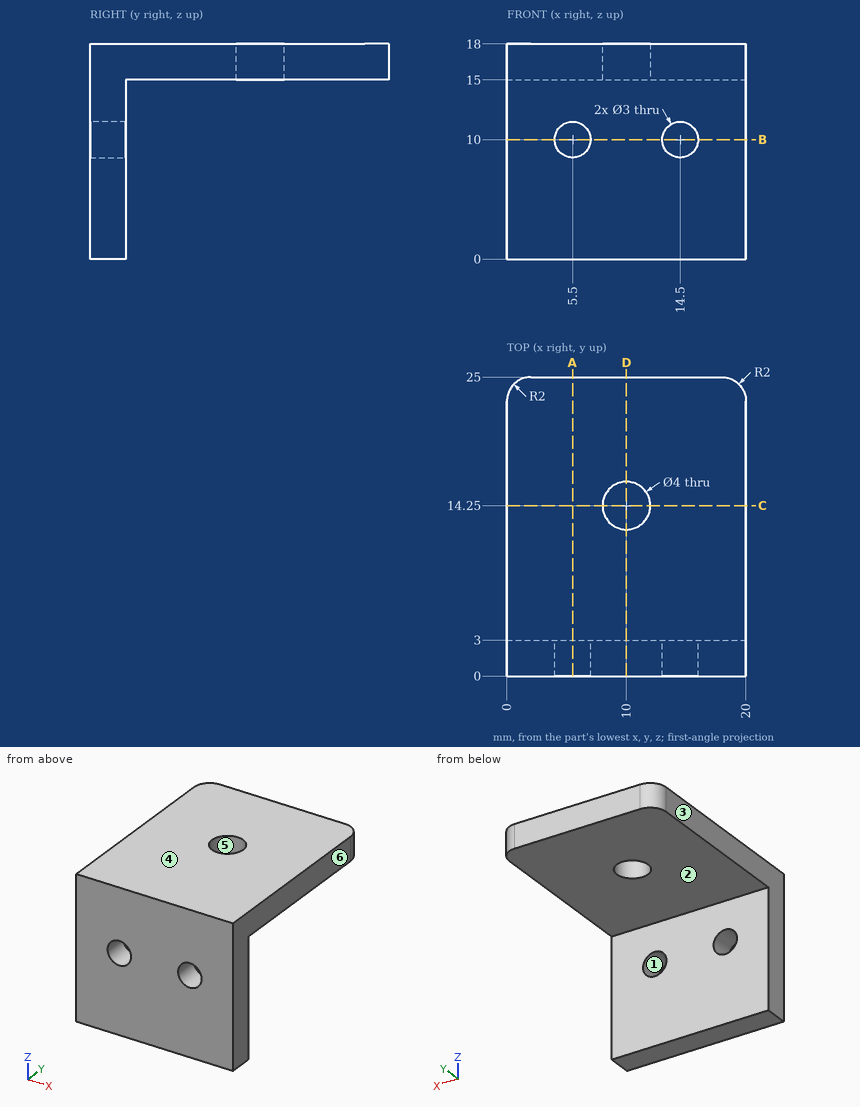
Can you work these out from the drawing? Everything is in mm from the part's minimum corner. A direction names the side the tool comes from. Round coordinates to 2 decimals unless told otherwise and drop trailing zeros. Order: outer loops, then holes, each group sorted by start corner. A loop starts at its lowest first (then second) coordinate and runs counter-clockwise, first axis right, second up. Notation, with made-up numbers: (61, -39) -> (90, -39) arc R26 cw to (90, -23) -> close; hole circle Ø10 at (1, 7). An arc over 180 degrees is marked (long way). Use CSV: the item, a comma, the result in double quotes.
1. I want a section at B-B on z = 10. List the corners of the cut face in (x, y) for me, and give its area (3 significant figures).
Recorded:
outline,"(0, 0) -> (4, 0) -> (4, 3) -> (0, 3) -> close; (7, 0) -> (13, 0) -> (13, 3) -> (7, 3) -> close; (16, 0) -> (20, 0) -> (20, 3) -> (16, 3) -> close"
area,"42.0 mm2"
2. Which directions (+Z, -Z, +X, -X, +Y, -Y) give clear straight access to the entire face, cutting with the end or side of a thin tool? Please do the marked faces 1 and 2.
Recorded:
face 1,"+Y, -Y"
face 2,"-Z, +X, -X, +Y"
3. I need wall thicknesses on line 1 along X through (y, z) = (2.25, 10); line 2 along Z through (x, y) = (16, 11.25); line 3 along Y through (x, z) = (3.75, 13.5). Which ranges of each line are inside material? Lowest first, please.
Recorded:
line 1,"x = 0 to 4, 7 to 13, 16 to 20"
line 2,"z = 15 to 18"
line 3,"y = 0 to 3"
4. I want a section at D-D on x = 10. List the corners of the cut face in (y, z) for me, and give its area (3 significant figures).
Recorded:
outline,"(0, 0) -> (3, 0) -> (3, 15) -> (12.25, 15) -> (12.25, 18) -> (0, 18) -> close; (16.25, 15) -> (25, 15) -> (25, 18) -> (16.25, 18) -> close"
area,"108 mm2"
5. Thinking about a two-plate mould opening in X: for the marked faces 3, 4, 5 and 6, which applies, pulls with the +X half, pulls with the -X half, needs draft (parallel to the pull), parting line crosses it, or undercut?
Recorded:
face 3,"pulls with the -X half"
face 4,"needs draft"
face 5,"undercut"
face 6,"pulls with the +X half"
6. I want a section at C-C on y = 14.25. List the corners of the cut face in (x, z) for me.
Recorded:
outline,"(0, 15) -> (8, 15) -> (8, 18) -> (0, 18) -> close; (12, 15) -> (20, 15) -> (20, 18) -> (12, 18) -> close"
7. I'm going to push flat-ended pins straight in: P1, Ø3.5, axis at x = 14.5, z = 10, coming from the +Y side; P2, Ø5, axis at x = 10, y = 14.25, coming from the -Z side. Where does each tip first touch, or does it pass through?
Recorded:
P1,"stops at y = 3"
P2,"stops at z = 15"
8. I want a section at A-A on x = 5.5. List the corners of the cut face in (y, z) for me.
Recorded:
outline,"(0, 0) -> (3, 0) -> (3, 8.5) -> (0, 8.5) -> close; (0, 11.5) -> (3, 11.5) -> (3, 15) -> (25, 15) -> (25, 18) -> (0, 18) -> close"
